Design review of the part built by this model. Coordinates are the model's own, in mm. Face numbers are marked on the shaded views. Coordinates: 2 decimals unless noted, no trailing zeros. Write each loop counter-clockwise with the first axis right and the second up, starting at its lowest first coordinate (ties: lowest second). Pieces come first, ordered by that corner, then holes.
Q1. To check wall thickness, follow probe 1 along X at (y, z) = (1.25, 18.5); probe 2 along X at (y, z) = (6.5, 6); probe 3 along Y at (x, z) = (-113.5, -73). State the ranges of each line that lie inside material, in increasing order.
Q2. Clearance check with flat-ended pins moving along their axes: pin 1 Ø1.5 at (x, y) = (-8.5, 3) entering from -Z; pin 2 Ø1.8 at (y, z) = (2, -40) entering from +X; pin 3 Ø4 at (y, z) = (5.5, -31) entering from -X. State where each tip first meets the part, or that it passes through.
Q3. Add section B-B, the plane z = 53. Give the boundary of the cut face in (x, y).
Q4. Add section C-C, the plane x = 8. Give the boundary of the cut face in (y, z), plus the area to 3 significant figures.
Q5. Add section A-A, the plane y = 4.25. Give the boundary of the cut face in (x, z), plus the area to 3 significant figures.
Q6. The part is to be moulded in two halves that separate along Y. For the marked faces 1 and 2, say which applies: +Y half, -Y half, draft (parallel to the pull), parting line (faces both ways), or undercut.
from build123d import *

# Parameters (mm, degrees)
SKETCH1_W           = 317
SKETCH1_H           = 182.5
BOSS_EXTRUDE1_DEPTH = 8
SKETCH3_W           = 22
SKETCH3_H           = 164.5
CUT_EXTRUDE3_DEPTH  = 184.065049914
SKETCH4_W           = 273
SKETCH4_H           = 164.5
CUT_EXTRUDE4_DEPTH  = 6
SKETCH5_W           = 20
SKETCH5_H           = 164.5
BOSS_EXTRUDE3_DEPTH = 6


with BuildPart() as part:
    # Sketch1 → Boss-Extrude1 (new body)
    with BuildSketch(Plane(origin=(0, 0, 0), x_dir=(1, 0, 0), z_dir=(0, 1, 0))):
        Rectangle(SKETCH1_W, SKETCH1_H)
    extrude(amount=BOSS_EXTRUDE1_DEPTH)

    # Sketch3 → Cut-Extrude3 (cut, through all)
    with BuildSketch(Plane(origin=(0, 8, 0), x_dir=(1, 0, 0), z_dir=(0, 1, 0))):
        with Locations((-147.5, 9)):
            Rectangle(SKETCH3_W, SKETCH3_H)
        with Locations((147.5, 9)):
            Rectangle(SKETCH3_W, SKETCH3_H)
    extrude(amount=-CUT_EXTRUDE3_DEPTH, mode=Mode.SUBTRACT)

    # Sketch4 → Cut-Extrude4 (cut)
    with BuildSketch(Plane.XZ):
        with Locations((0, -9)):
            Rectangle(SKETCH4_W, SKETCH4_H)
    extrude(amount=-CUT_EXTRUDE4_DEPTH, mode=Mode.SUBTRACT)

    # Sketch5 → Boss-Extrude3 (add)
    with BuildSketch(Plane.XZ.offset(-6)):
        with Locations((-126.5, -9)):
            Rectangle(SKETCH5_W, SKETCH5_H)
        with Locations((126.5, -9)):
            Rectangle(SKETCH5_W, SKETCH5_H)
    extrude(amount=BOSS_EXTRUDE3_DEPTH)


solid = part.part
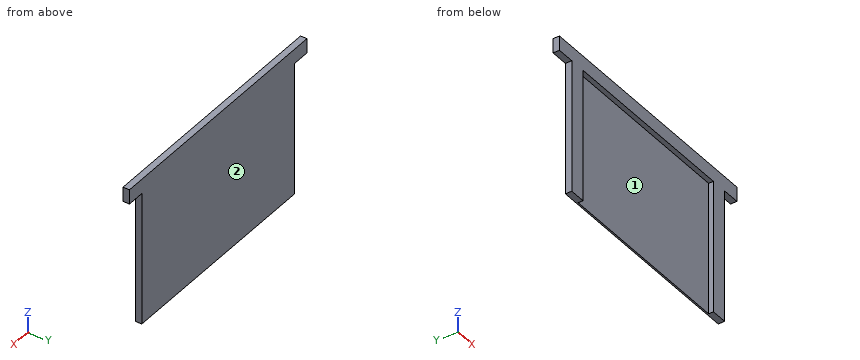
Here are the results:
1. probe 1: x = -136.5 to -116.5, 116.5 to 136.5
1. probe 2: x = -136.5 to 136.5
1. probe 3: y = 6 to 8
2. pin 1: stops at z = 73.25
2. pin 2: stops at x = 136.5
2. pin 3: stops at x = -136.5
3. outline: (-136.5, 0) - (-116.5, 0) - (-116.5, 6) - (116.5, 6) - (116.5, 0) - (136.5, 0) - (136.5, 8) - (-136.5, 8) - close
4. outline: (0, 73.25) - (6, 73.25) - (6, -91.25) - (8, -91.25) - (8, 91.25) - (0, 91.25) - close
4. area: 473 mm2
5. outline: (-158.5, 73.25) - (-136.5, 73.25) - (-136.5, -91.25) - (-116.5, -91.25) - (-116.5, 73.25) - (116.5, 73.25) - (116.5, -91.25) - (136.5, -91.25) - (136.5, 73.25) - (158.5, 73.25) - (158.5, 91.25) - (-158.5, 91.25) - close
5. area: 12,300 mm2
6. face 1: -Y half
6. face 2: +Y half
